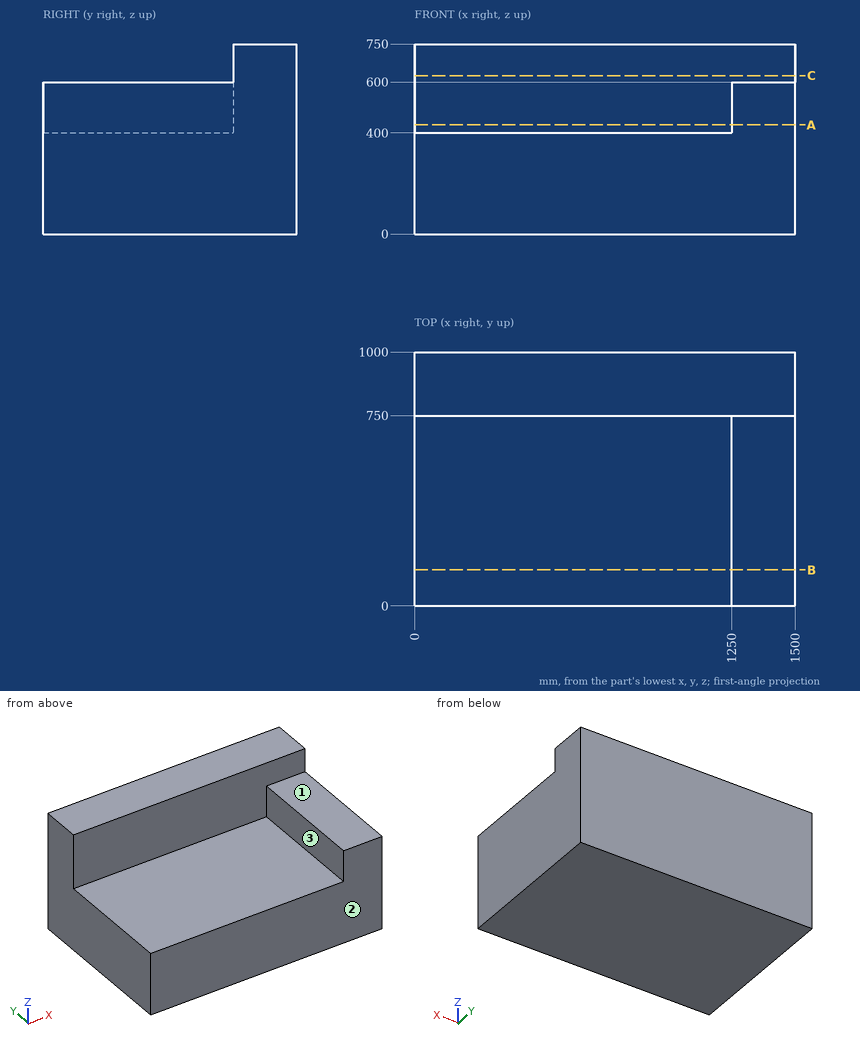
Could you check a few things on this drawing? It's one solid part, dimensions in mm from its lowest x, y, z. A direction names the side the tool comes from. Round coordinates to 2 decimals unless told otherwise and drop trailing zeros. Order: outer loops, then holes, each group sorted by start corner. A loop starts at its lowest first (then second) coordinate and runs counter-clockwise, first axis right, second up. Notation, with made-up numbers: M -29,-9 L 25,-9 A22 ccw 25,26 Z; hole C 29,0.25 d5. An arc over 180 degrees is marked long. Return JSON: item names as keys, results as strings. Group by question number.
1. Please list where these lines run through material, in increasing order: probe 1 along Z at (x, y) = (1123.5, 348.5); probe 2 along Y at (x, z) = (1058, 635.5); probe 3 along X at (y, z) = (466.5, 471).
2. If we section it at C-C on z = 625.5: List the corners of the cut face in (x, y) for me.
3. I'm going to push a flat-ended pin straight in: pin 1 Ø4 at (x, y) = (973, 430.5) entering from -Z. Where does the tip first touch, or does it pass through?
4. On a 3-axis mill with a long thin cutter (end or side, diameter ignored), from which of +Z, -Z, +X, -X, +Y, -Y can I reach the whole of each face in a straight line? I mean the marked faces 1, 2 and 3. Say none if no direction works.
5. If we section it at A-A on z = 431.5: List the corners of the cut face in (x, y) for me, then the cut area to 4 significant figures.
6. If we section it at B-B on y = 142: List the corners of the cut face in (x, z) for me.
Reply:
{
 "1": {"probe 1": "0 to 400", "probe 2": "750 to 1000", "probe 3": "1250 to 1500"},
 "2": {"outline": "M 0,750 L 1500,750 L 1500,1000 L 0,1000 Z"},
 "3": {"pin 1": "z = 0"},
 "4": {"face 1": "+Z, +X, -X, -Y", "face 2": "+Z, -Z, +X, -X, -Y", "face 3": "+Z, -X, -Y"},
 "5": {"outline": "M 0,750 L 1250,750 L 1250,0 L 1500,0 L 1500,1000 L 0,1000 Z", "area": "562,500 mm^2"},
 "6": {"outline": "M 0,0 L 1500,0 L 1500,600 L 1250,600 L 1250,400 L 0,400 Z"}
}
